The listing builds one solid part. Answer for the finished solid, in the listing's coordinates (mm). A direction names the side the tool comes from. Give positions to 0.01 mm unless a question says otherwise; leave off trailing zeros. Write each loop counter-clockwise with the first axis right and the second up, starting at its lowest first coordinate (ties: lowest second). Pieces come first, ordered by that corner, then holes. Notation, with made-up numbers: M 44.25,-20.75 L 99.25,-20.75 A33 ccw 99.25,9.25 Z; hole C -31.5,28.25 d6. An arc over 180 degrees is marked long. Answer as a JSON object with one key per item and string values.
```python
from build123d import *

# Parameters (mm, degrees)
SKETCH1_W                 = 38.735
SKETCH1_H                 = 4.7625
F_8_32_TAPPED_HOLE1_D     = 3.4544
F_8_32_TAPPED_HOLE1_DEPTH = 10.7188
F_8_32_TAPPED_HOLE1_TIP   = 1.037806461
F_8_32_TAPPED_HOLE2_D     = 3.4544
F_8_32_TAPPED_HOLE2_DEPTH = 10.7188
F_8_32_TAPPED_HOLE2_TIP   = 1.037806461


with BuildPart() as part:
    # Sketch1 → Revolve1 (revolve)
    with BuildSketch(Plane(origin=(0, 0, 0), x_dir=(0, 0, -1), z_dir=(1, 0, 0)), mode=Mode.PRIVATE) as revolve1_sk:
        with Locations((19.3675, 2.38125)):
            Rectangle(SKETCH1_W, SKETCH1_H)
    revolve(revolve1_sk.sketch.rotate(Axis((0, 0, 0), (0, 0, 1)), 90), axis=Axis((0, 0, 0), (0, 0, 1)))

    # 8-32 Tapped Hole1
    with Locations(Plane.XY):
        with Locations((0, 0)):
            Hole(F_8_32_TAPPED_HOLE1_D / 2, depth=F_8_32_TAPPED_HOLE1_DEPTH)
            with Locations((0, 0, -(F_8_32_TAPPED_HOLE1_DEPTH + F_8_32_TAPPED_HOLE1_TIP / 2))):  # 118° drill point
                Cone(0, F_8_32_TAPPED_HOLE1_D / 2, F_8_32_TAPPED_HOLE1_TIP, mode=Mode.SUBTRACT)

    # 8-32 Tapped Hole2
    with Locations(Plane(origin=(0, 0, -38.735), x_dir=(-1, 0, 0), z_dir=(0, 0, -1))):
        with Locations((0, 0)):
            Hole(F_8_32_TAPPED_HOLE2_D / 2, depth=F_8_32_TAPPED_HOLE2_DEPTH)
            with Locations((0, 0, -(F_8_32_TAPPED_HOLE2_DEPTH + F_8_32_TAPPED_HOLE2_TIP / 2))):  # 118° drill point
                Cone(0, F_8_32_TAPPED_HOLE2_D / 2, F_8_32_TAPPED_HOLE2_TIP, mode=Mode.SUBTRACT)


solid = part.part
```
1. A cutting plane is placed at B-B, the plane z = -14.5. Give the vertices of the cut face in (x, y) (1 decimal), plus the area to 3 significant figures.
Verdict:
{"outline": "C 0,0 d9.5", "area": "71.3 mm2"}
2. A cutting plane is placed at C-C, the plane y = -2.75. Give the vertices of the cut face in (x, z) (3 decimals).
Verdict:
{"outline": "M -3.888,-38.735 L 3.888,-38.735 L 3.888,0 L -3.888,0 Z"}
3. The mould has two halves that part along X. Classify faces 3 (the flat face through (2, 0, -38.735)), 4 (the conical face through (0.277, -0.115, -11.576)), 5 (the cylindrical face through (0.225, 1.713, -5.434)), 6 (the cylindrical face through (1.03, 4.65, -19.64)): released by +X, released by -X, zero draft, split by the parting line, or undercut.
Verdict:
{"face 3": "zero draft", "face 4": "undercut", "face 5": "undercut", "face 6": "split by the parting line"}
4. Flat-ended cylindrical pins translate along their axes: pin 1 (3 mm diameter, centred on y = -0.5, z = -24, fed in from -X); pin 2 (3 mm diameter, centred on x = 0, y = 0, fed in from -Z). Find the tip coordinate at first contact, or state that the pin passes through.
Verdict:
{"pin 1": "stops at x = -4.76", "pin 2": "stops at z = -27.88"}
5. A cutting plane is placed at A-A, the plane z = -30.5. Give the vertices of the cut face in (x, y) (1 decimal), plus the area to 3 significant figures.
Verdict:
{"outline": "C 0,0 d9.5; hole C 0,0 d3.5", "area": "61.9 mm2"}
6. A cutting plane is placed at D-D, the plane x = 3.25. Give the vertices of the cut face in (y, z) (3 decimals).
Verdict:
{"outline": "M -3.481,-38.735 L 3.481,-38.735 L 3.481,0 L -3.481,0 Z"}
7. For faces 1 (the flat face through (2, 0, 0)), 2 (the cylindrical face through (-0.225, 1.713, -33.301)), determine the directions among +Z, -Z, +X, -X, +Y, -Y from which every point of the face is accessible in a straight line to the end or side of a thin tool.
Verdict:
{"face 1": "+Z, +X, -X, +Y, -Y", "face 2": "-Z"}
8. Consider line 1 along Y through (x, z) = (0, -36.25); line 2 along X through (y, z) = (1.5, -35); line 3 along Y through (x, z) = (-1.25, -2.5). Determine where each line is inside the solid, lowest interval first.
Verdict:
{"line 1": "y = -4.76 to -1.73, 1.73 to 4.76", "line 2": "x = -4.52 to -0.86, 0.86 to 4.52", "line 3": "y = -4.6 to -1.19, 1.19 to 4.6"}
